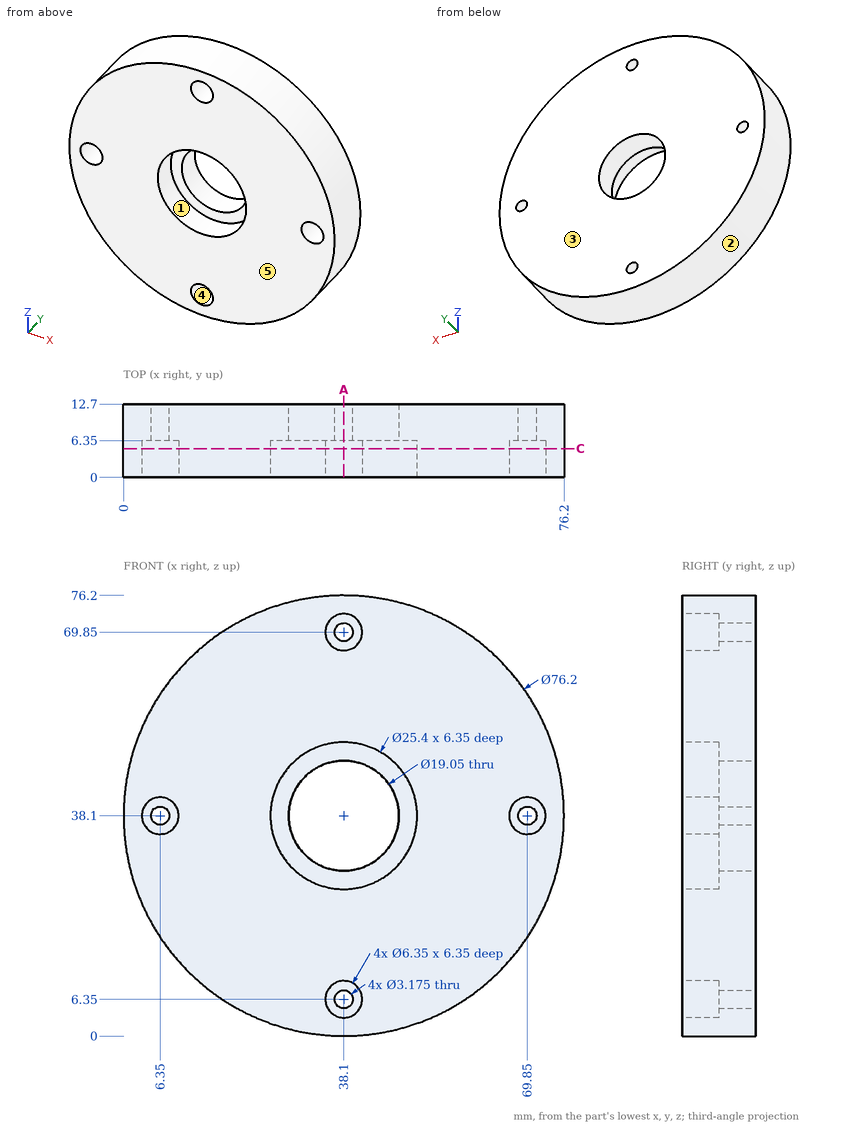
Can you work these out from the drawing? Everything is in mm from the part's minimum corner. A direction names the side the tool comes from. Give positions to 0.01 mm unless a question says otherwise; leave off trailing zeros. Loops run counter-clockwise (first coordinate to the right, second up) from the corner with the lowest first, then second, coordinate; pieces in that order, holes last. Notation, with made-up numbers: (21.25, 0) - (72.25, 0) arc R26 ccw to (72.25, 31) - close; hole circle Ø10 at (5.25, -18.75). An arc over 180 degrees is marked (long way). Answer as a JSON object with one key per item and string values.
Q1. If we mould it in two halves opening along Z, with no side actions, what happens to the marked faces 1, 2 and 3? For each: pulls with the +Z half, pulls with the -Z half, needs draft (parallel to the pull), parting line crosses it, or undercut.
Geometry says:
{"face 1": "undercut", "face 2": "parting line crosses it", "face 3": "needs draft"}
Q2. Will these pins go through, and if not, where does the flat tip stop? P1, Ø3.5, axis at x = 6.35, z = 38.1, coming from the -Y side; P2, Ø1, axis at x = 40, y = 9, coming from the +Z side; P3, Ø5, axis at x = 52, y = 1.5, coming from the -Z side.
Geometry says:
{"P1": "y = 6.35", "P2": "z = 76.17", "P3": "z = 1.75"}
Q3. Imagine slicing it at A-A on x = 38.1. Give the number of separate pieces and of enclosed holes in the cut face, plus the area to 3 significant figures.
Geometry says:
{"separate pieces": "4", "enclosed holes": "0", "area": "565 mm²"}
Q4. If I drill on L1, parallel to Z at x = 38.1, y = 8 (1 decimal); L2, parallel to Z at x = 38.1, y = 1.75 (3 decimals); L3, parallel to X at y = 5.25, z = 31, over which ranges is the centre line in solid material (lowest first)?
Geometry says:
{"L1": "0 to 4.8, 7.9 to 28.6, 47.6 to 68.3, 71.4 to 76.2", "L2": "0 to 3.175, 9.525 to 25.4, 50.8 to 66.675, 73.025 to 76.2", "L3": "0.67 to 27.57, 48.63 to 75.53"}
Q5. Imagine slicing it at C-C on y = 5. Write out the boundary of the cut face in (x, z) (3 decimals), plus the area to 3 significant figures.
Geometry says:
{"outline": "circle Ø76.2 at (38.1, 38.1); hole circle Ø6.35 at (6.35, 38.1); hole circle Ø25.4 at (38.1, 38.1); hole circle Ø6.35 at (38.1, 6.35); hole circle Ø6.35 at (38.1, 69.85); hole circle Ø6.35 at (69.85, 38.1)", "area": "3,930 mm²"}
Q6. Which directions (+Z, -Z, +X, -X, +Y, -Y) give clear straight access to the entire face, cutting with the end or side of a thin tool? Please do the marked faces 4 and 5.
Geometry says:
{"face 4": "-Y", "face 5": "+Z, -Z, +X, -X, -Y"}
